Autodesk Inventor part; units mm, degrees
ref_plane "YZ Plane" through (0, 0, 0) normal (1, 0, 0) x (0, 1, 0)
ref_plane "XZ Plane" through (0, 0, 0) normal (0, 1, 0) x (-1, 0, 0)
ref_plane "XY Plane" through (0, 0, 0) normal (0, 0, 1) x (1, 0, 0)
sketch "Sketch1" plane through (0, 0, 0) normal (0, 1, 0) x (-1, 0, 0)
  line L0 (0, 0) -> (6, 0)
  line L1 (6, 0) -> (6, -41)
  line L2 (6, -41) -> (0, -41)
  line L3 (0, -41) -> (0, 0)
  line L4 (7, -42) -> (7, 1)
  line L5 (7, 1) -> (-1, 1)
  line L6 (-1, 1) -> (-1, -42)
  line L7 (-1, -42) -> (7, -42)
  line L8 (3, 1) -> (3, 3)
  circle A0 centre (3, 3) radius 1.5
  arc A1 (7, 3) -> (-1, 3) centre (3, 3) ccw
  line L9 (7, 1) -> (7, 3)
  line L10 (-1, 1) -> (-1, 3)
  line L11 (3, -42) -> (3, -44)
  circle A2 centre (3, -44) radius 1.5
  arc A3 (-1, -44) -> (7, -44) centre (3, -44) ccw
  line L12 (7, -42) -> (7, -44)
  line L13 (-1, -42) -> (-1, -44)
  dimension "d19" = 2
  dimension "d0" = 6
  dimension "d1" = 41
  dimension "d2" = 1
  dimension "d3" = 2
  dimension "d4" = 3
  dimension "d5" = 8
  dimension "d6" = 2
  dimension "d7" = 3
  dimension "d8" = 8
extrude "Extrusion1" add sketch "Sketch1" along normal blind 3
sketch "Sketch2" plane through (0, 3, 0) normal (0, 1, 0) x (1, 0, 0)
  line L0 (0, 41) -> (0, 0)
  line L1 (-6, 0) -> (-6, 41)
  line L2 (0, 0) -> (-6, 0)
  line L3 (-6, 0) -> (-6, 41)
  line L4 (-6, 41) -> (0, 41)
  line L5 (0, 41) -> (0, 0)
extrude "Extrusion2" add sketch "Sketch2" against normal blind 1
sketch "Sketch3" plane through (0, 0, 0) normal (0, -1, 0) x (1, 0, 0)
  circle A0 centre (-3, 3) radius 1.5
  line L0 (-6, -41) -> (-6, 0)
  line L1 (-6, 0) -> (0, 0)
  line L2 (0, 0) -> (0, -41)
  line L3 (0, -41) -> (-6, -41)
  circle A1 centre (-3, 3) radius 1.5
  circle A2 centre (-3, -44) radius 1.5
  line L4 (-7, -44) -> (-7, 3)
  arc A3 (-7, -44) -> (1, -44) centre (-3, -44) ccw
  line L5 (1, 3) -> (1, -44)
  arc A4 (1, 3) -> (-7, 3) centre (-3, 3) ccw
  line L6 (-7, -44) -> (-7, 3)
  line L7 (-7, -20.5) -> (-7, -21.5)
  line L8 (-7, -21.5) -> (-6, -21.5)
  line L9 (-6, -21.5) -> (-6, -19.5)
  line L10 (-6, -19.5) -> (-7, -19.5)
  line L11 (-7, -19.5) -> (-7, -21.5)
  dimension "d13" = 1
  dimension "d14" = 1
  dimension "d15" = 2
extrude "Extrusion3" cut sketch "Sketch3" against normal up to surface (2 mm away) contours L8 L4 L10 L0
chamfer "Chamfer1" distance 1 angle 45 2 edges at (-6.5, 0, -19.5) (-6.5, 0, -21.5)
chamfer "Chamfer2" distance 1 angle 45 2 edges at (-3, 0, 0) (-3, 0, -41)
properties part number "Beaglebone Antenna Mount"
CAD build for the part. Positions are in the model's coordinates, mm. A direction names the side the tool comes from. Round coordinates to 2 decimals unless told otherwise and drop trailing zeros. Loops run counter-clockwise (first coordinate to the right, second up) from the corner with the lowest first, then second, coordinate; pieces in that order, holes last. Notation, with made-up numbers: M -22,-5 L 1,-5 A27 cw 1,20 Z; hole C 54,81.25 d2. An arc over 180 degrees is marked long. Return JSON: item names as keys, results as strings. Group by question number.
(1) Saw through at B-B, the plane y = 2.5. List the corners of the cut face in (x, z), and give its area (3 significant figures).
(2) Drop flat-ended pins along their axis: P1, Ø0.5, axis at x = -2, y = 1.5, coming from the -Z side; P2, Ø0.8, axis at x = -6.5, y = 1.5, coming from the +Z side; P3, Ø1.1, axis at x = -6.5, y = 1.5, coming from the -Z side. Give the stop position or say it passes through.
(3) Saw through at D-D, the plane z = -43. List the corners of the cut face in (x, y), and give its area (3 significant figures).
(4) Wall check: probe 1 along Z at (x, y) = (-3, 1.15); probe 2 along X at (y, z) = (1.75, 3); probe 3 along X at (y, z) = (0.55, -30). Give the ranges that are in metal, low to high. Write a range as [from, to].
(5) Saw through at C-C, the plane z = -4. List the corners of the cut face in (x, y), and give its area (3 significant figures).
(6) Mould opens along Z. For faces 1 (the flat face through (-6.5, 1.5, -21.5)), 2 (the flat face through (1, 1, -20)) say: +Z half, -Z half, draft (parallel to the pull), parting line (faces both ways), or undercut.
(7) Tool access for faces 3 (the cylindrical face through (-2.675, 1.479, -42.536)), 4 (the flat face through (-6.5, 0.5, -22)), 5 (the flat face through (-3, 1.5, 0)): list every direction of +Z, -Z, +X, -X, +Y, -Y with a clear straight run to the whole face (end or side of a thin tool).
(8) Saw through at A-A, the plane x = -3. List the corners of the cut face in (y, z).
Answer list:
{
 "1": {"outline": "M -7,-44 A4 ccw 1,-44 L 1,3 A4 ccw -7,3 Z; hole C -3,-44 d3; hole C -3,3 d3", "area": "412 mm2"},
 "2": {"P1": "z = -47.93", "P2": "z = 5.53", "P3": "z = -46.7"},
 "3": {"outline": "M -7,0 L -4.12,0 L -4.12,3 L -7,3 Z; M -1.88,0 L 1,0 L 1,3 L -1.88,3 Z", "area": "17.3 mm2"},
 "4": {"probe 1": "[-48, -45.5], [-42.5, -41], [0, 1.5], [4.5, 7]", "probe 2": "[-7, -4.5], [-1.5, 1]", "probe 3": "[-7, -6], [0, 1]"},
 "5": {"outline": "M -7,0 L -6,0 L -6,2 L 0,2 L 0,0 L 1,0 L 1,3 L -7,3 Z", "area": "12.0 mm2"},
 "6": {"face 1": "undercut", "face 2": "draft"},
 "7": {"face 3": "+Y, -Y", "face 4": "-X, -Y", "face 5": "-Y"},
 "8": {"outline": "M 0,-48 L 3,-48 L 3,-45.5 L 0,-45.5 Z; M 0,-42.5 L 3,-42.5 L 3,1.5 L 0,1.5 L 0,1 L 1,0 L 2,0 L 2,-41 L 1,-41 L 0,-42 Z; M 0,4.5 L 3,4.5 L 3,7 L 0,7 Z"}
}
